The model under review builds one solid part; all positions refer to its coordinate system, in mm. Face numbers are marked on the shaded views. A direction names the side the tool comes from. Give positions to 0.01 mm unless a question says otherwise; leave off trailing zeros. Order: outer loops, then holes, each group sorted by start corner. A loop starts at its lowest first (then second) coordinate and runs counter-clockwise, first axis right, second up. Notation, with made-up numbers: M 54,-26 L 89,-26 A13 ccw 89,-10 Z; hole C -16,86 d6. An arc over 180 degrees is marked long. One line per question, with ' | ' between items. Start each with the question number.
1. We need section D-D on z = 0. Write out the cut boundary in (x, y).
2. We need section B-B on x = -9.5. Write out the cut boundary in (y, z).
3. We need section C-C on y = 2.1. Write out the cut boundary in (x, z), then the cut area to 3 significant figures.
4. Insertion check: P1, Ø1, axis at x = 1, y = 3.5, coming from the +Z side; P2, Ø2, axis at x = -9, z = 5.5, coming from the +Y side; P3, Ø0.6, axis at y = 3, z = -0.5, coming from the -X side; P4, Ø3, axis at x = -9, z = -5.5, coming from the +Y side. Each pin has a flat end and moves straight along its axis. Give the tip position at first contact, or say it passes through.
5. Wall thickness on L1, parallel to X at y = 0.9, z = -5.5; L2, parallel to Z at x = -9, y = 1.3; L3, parallel to Y at x = 10, z = 11.25: over which ranges is each line inside the solid? List them lowest first.
6. We need section A-A on z = -5.5. Write out the cut boundary in (x, y).
7. The part is to be moulded in two halves that separate along Z. For the marked faces 1 and 2, say which applies: +Z half, -Z half, draft (parallel to the pull), parting line (faces both ways), or undercut.
8. For the marked faces 3 and 4, list the 3-axis set-ups (+Z, -Z, +X, -X, +Y, -Y) from which the entire face can be reached by the end or side of a thin tool; tool diameter is ignored.
```python
from build123d import *

# Parameters (mm, degrees)
SKETCH1_W                 = 22
SKETCH1_H                 = 15
BOSS_EXTRUDE1_DEPTH       = 2.5
F_1_0MM_DOWEL_HOLE1_D     = 2.6
F_1_0MM_DOWEL_HOLE1_DEPTH = 6.35
F_1_0MM_DOWEL_HOLE1_TIP   = 0.781118805
SKETCH4_W                 = 5
SKETCH4_H                 = 4.4
BOSS_EXTRUDE2_DEPTH       = 1.2
SKETCH5_W                 = 22
SKETCH5_H                 = 13
BOSS_EXTRUDE3_DEPTH       = 2.5
SKETCH6_W                 = 8.928834932
SKETCH6_H                 = 2.022342955
BOSS_EXTRUDE4_DEPTH       = 2
SKETCH7_R                 = 1.677550445
BOSS_EXTRUDE5_DEPTH       = 0.25


with BuildPart() as part:
    # Sketch1 → Boss-Extrude1 (new body)
    with BuildSketch(Plane(origin=(0, 0, 0), x_dir=(1, 0, 0), z_dir=(0, 1, 0))):
        Rectangle(SKETCH1_W, SKETCH1_H)
    extrude(amount=BOSS_EXTRUDE1_DEPTH)

    # Ø1.0mm Dowel Hole1
    with Locations(Plane(origin=(0, 2.5, 0), x_dir=(1, 0, 0), z_dir=(0, 1, 0))):
        with Locations((-9, 5.5), (9, 5.5), (9, -5.5), (-9, -5.5)):
            Hole(F_1_0MM_DOWEL_HOLE1_D / 2, depth=F_1_0MM_DOWEL_HOLE1_DEPTH)
            with Locations((0, 0, -(F_1_0MM_DOWEL_HOLE1_DEPTH + F_1_0MM_DOWEL_HOLE1_TIP / 2))):  # 118° drill point
                Cone(0, F_1_0MM_DOWEL_HOLE1_D / 2, F_1_0MM_DOWEL_HOLE1_TIP, mode=Mode.SUBTRACT)

    # Sketch4 → Boss-Extrude2 (add)
    with BuildSketch(Plane(origin=(0, 2.5, 0), x_dir=(1, 0, 0), z_dir=(0, 1, 0))):
        Rectangle(SKETCH4_W, SKETCH4_H)
    extrude(amount=BOSS_EXTRUDE2_DEPTH)

    # Sketch5 → Boss-Extrude3 (add)
    with BuildSketch(Plane(origin=(0, 2.5, 0), x_dir=(1, 0, 0), z_dir=(0, 1, 0))):
        with Locations((0, -14)):
            Rectangle(SKETCH5_W, SKETCH5_H)
    extrude(amount=-BOSS_EXTRUDE3_DEPTH)

    # Sketch6 → Boss-Extrude4 (add)
    with BuildSketch(Plane(origin=(0, 2.5, 0), x_dir=(1, 0, 0), z_dir=(0, 1, 0))):
        with Locations((-0.152629657, -13.139390077)):
            Rectangle(SKETCH6_W, SKETCH6_H)
    extrude(amount=BOSS_EXTRUDE4_DEPTH)

    # Sketch7 → Boss-Extrude5 (add)
    with BuildSketch(Plane(origin=(0, 3.7, 0), x_dir=(1, 0, 0), z_dir=(0, 1, 0))):
        Circle(SKETCH7_R)
    extrude(amount=BOSS_EXTRUDE5_DEPTH)


solid = part.part
```
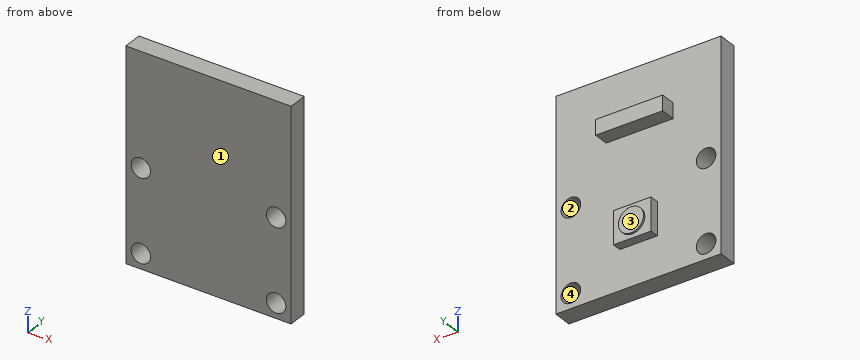
Entries:
1) outline: M -11,0 L 11,0 L 11,2.5 L 2.5,2.5 L 2.5,3.7 L 1.68,3.7 L 1.68,3.95 L -1.68,3.95 L -1.68,3.7 L -2.5,3.7 L -2.5,2.5 L -11,2.5 Z
2) outline: M 0,-7.5 L 2.5,-7.5 L 2.5,-6.7 L 0,-6.7 Z; M 0,-4.3 L 2.5,-4.3 L 2.5,4.3 L 0,4.3 Z; M 0,6.7 L 2.5,6.7 L 2.5,20.5 L 0,20.5 Z
3) outline: M -11,-7.5 L 11,-7.5 L 11,20.5 L -11,20.5 Z; hole C -9,-5.5 d2.6; hole C -9,5.5 d2.6; hole C 9,-5.5 d2.6; hole C 9,5.5 d2.6 | area: 595 mm^2
4) P1: stops at z = 14.15 | P2: passes through | P3: stops at x = -2.5 | P4: stops at y = 2.5
5) L1: x = -11 to -10.3, -7.7 to 7.7, 10.3 to 11 | L2: z = -7.5 to -6.8, -4.2 to 4.2, 6.8 to 20.5 | L3: y = 0 to 2.5
6) outline: M -11,0 L -10.3,0 L -10.3,2.5 L -11,2.5 Z; M -7.7,0 L 7.7,0 L 7.7,2.5 L -7.7,2.5 Z; M 10.3,0 L 11,0 L 11,2.5 L 10.3,2.5 Z
7) face 1: draft | face 2: undercut
8) face 3: -Z, +X, -X, +Y | face 4: +Y, -Y
